Part model, mm, in its own coordinate system. A direction names the side the tool comes from. Give positions to 0.01 mm unless a question says otherwise; leave off trailing zeros. Order: outer loops, then holes, each group sorted by start corner. A loop starts at its lowest first (then second) coordinate and runs counter-clockwise, first axis right, second up. Notation, with made-up numbers: (-4, -10) - (28, -10) arc R19 cw to (28, -5) - close; hole circle Ø2 at (4, 43.5). An arc over 180 degrees is marked (long way). Use a Markdown table: item, result. Add a question column.
from build123d import *

# Parameters (mm, degrees)
BOSS_EXTRUDE1_DEPTH = 152.4
CUT_EXTRUDE1_REACH  = 17.875
SKETCH3_R           = 3.2512
CUT_EXTRUDE2_START  = -275.7932
CUT_EXTRUDE2_DEPTH  = 275.7932
CUT_EXTRUDE3_REACH  = 17.875
SKETCH5_R           = 1.5875


with BuildPart() as part:
    # Sketch2 → Boss-Extrude1 (new body, symmetric)
    with BuildSketch(Plane.XY):
        with BuildLine():
            Line((-7.9375, 0), (7.9375, 0))
            Line((7.9375, 0), (7.9375, 15.875))
            Line((7.9375, 15.875), (7.14375, 15.875))
            ThreePointArc((7.14375, 15.875), (6.582483992, 15.642516008), (6.35, 15.08125))
            Line((6.35, 15.08125), (6.35, 2.38125))
            ThreePointArc((6.35, 2.38125), (6.117516008, 1.819983992), (5.55625, 1.5875))
            Line((5.55625, 1.5875), (-7.14375, 1.5875))
            ThreePointArc((-7.14375, 1.5875), (-7.705016008, 1.355016008), (-7.9375, 0.79375))
            Line((-7.9375, 0.79375), (-7.9375, 0))
        make_face()
    extrude(amount=BOSS_EXTRUDE1_DEPTH, both=True)

    # Sketch3 → Cut-Extrude1 (cut, up to next)
    with BuildSketch(Plane(origin=(7.9375, 0, 0), x_dir=(0, 0, -1), z_dir=(1, 0, 0)), mode=Mode.PRIVATE) as cut_extrude1_sk1:
        with Locations((144.907, 10.7061)):
            Circle(SKETCH3_R)
    cut_extrude1_tool1 = extrude(cut_extrude1_sk1.sketch, amount=-CUT_EXTRUDE1_REACH, mode=Mode.PRIVATE) & part.part
    add(cut_extrude1_tool1.solids().sort_by_distance((7.9375, 10.7061, -144.907))[0], mode=Mode.SUBTRACT)
    # Sketch3 → Cut-Extrude1 (cut, up to next)
    with BuildSketch(Plane(origin=(7.9375, 0, 0), x_dir=(0, 0, -1), z_dir=(1, 0, 0)), mode=Mode.PRIVATE) as cut_extrude1_sk2:
        with Locations((130.9116, 10.7061)):
            Circle(SKETCH3_R)
    cut_extrude1_tool2 = extrude(cut_extrude1_sk2.sketch, amount=-CUT_EXTRUDE1_REACH, mode=Mode.PRIVATE) & part.part
    add(cut_extrude1_tool2.solids().sort_by_distance((7.9375, 10.7061, -130.9116))[0], mode=Mode.SUBTRACT)

    # Sketch4 → Cut-Extrude2 (cut)
    with BuildSketch(Plane.XY.offset(152.4).offset(CUT_EXTRUDE2_START)):
        with BuildLine():
            Line((-7.9375, 0.79375), (-7.9375, 0))
            Line((-7.9375, 0), (7.9375, 0))
            Line((7.9375, 0), (7.9375, 15.875))
            Line((7.9375, 15.875), (7.14375, 15.875))
            ThreePointArc((7.14375, 15.875), (6.582483992, 15.642516008), (6.35, 15.08125))
            Line((6.35, 15.08125), (6.35, 2.38125))
            ThreePointArc((6.35, 2.38125), (6.117516008, 1.819983992), (5.55625, 1.5875))
            Line((5.55625, 1.5875), (-7.14375, 1.5875))
            ThreePointArc((-7.14375, 1.5875), (-7.705016008, 1.355016008), (-7.9375, 0.79375))
        make_face()
    extrude(amount=CUT_EXTRUDE2_DEPTH, mode=Mode.SUBTRACT)

    # Sketch5 → Cut-Extrude3 (cut, up to next)
    with BuildSketch(Plane.XZ, mode=Mode.PRIVATE) as cut_extrude3_sk1:
        with Locations((0, -137.8966)):
            Circle(SKETCH5_R)
    cut_extrude3_tool1 = extrude(cut_extrude3_sk1.sketch, amount=-CUT_EXTRUDE3_REACH, mode=Mode.PRIVATE) & part.part
    add(cut_extrude3_tool1.solids().sort_by_distance((0, 0, -137.8966))[0], mode=Mode.SUBTRACT)


solid = part.part
1. Cut at D-D (y = 6.5). Write the cut outline in (x, z).
2. Tool access for faces 4 (the face through (2, 0, -138)), 5 (the face through (-2, 1.588, -138)): list every direction of +Z, -Z, +X, -X, +Y, -Y with a clear straight run to the whole face (end or side of a thin tool).
3. Cut at A-A (x = 0). Write the cut outline in (y, z), plus the area to 3 significant figures.
4. Pin check, flat tips, straight feed: P1, Ø6, axis at x = 2.5, z = -147, coming from the +Y side; P2, Ø8.5, axis at y = 10.71, z = -144.91, coming from the +X side; P3, Ø8, axis at y = 10.5, z = -126.5, coming from the -X side; P4, Ø1.9, axis at x = 0, z = -137.9, coming from the -Y side (3 decimals). Stop position of each tip, or through.
5. Drill centre lines: probe 1 along Z at (x, y) = (6.75, 10.25); probe 2 along X at (y, z) = (13.75, -140); probe 3 along Y at (x, z) = (2.5, -131.5). Where is each one in solid material? Low to high. Write a range as [from, to].
6. Mould opens along X. For faces 1 (the face through (-0.344, 0.783, -139.446)), 2 (the face through (7.155, 13.448, -132.659)), 3 (the face through (6.35, 9, -138)) say: released by +X, released by -X, zero draft, split by the parting line, or undercut.
Responses:
| question | item | result |
|---|---|---|
| 1 | outline | (6.35, -152.4) - (7.94, -152.4) - (7.94, -123.39) - (6.35, -123.39) - close |
| 2 | face 4 | +Z, -Z, +X, -X, -Y |
| 2 | face 5 | +Z, -Z, -X, +Y |
| 3 | outline | (0, -152.4) - (1.59, -152.4) - (1.59, -139.48) - (0, -139.48) - close; (0, -136.31) - (1.59, -136.31) - (1.59, -123.39) - (0, -123.39) - close |
| 3 | area | 41.0 mm² |
| 4 | P1 | stops at y = 1.59 |
| 4 | P2 | stops at x = 7.94 |
| 4 | P3 | stops at x = 6.35 |
| 4 | P4 | passes through |
| 5 | probe 1 | z = [-152.4, -148.13], [-141.69, -134.13], [-127.69, -123.39] |
| 5 | probe 2 | x = [6.35, 7.94] |
| 5 | probe 3 | y = [0, 1.59] |
| 6 | face 1 | undercut |
| 6 | face 2 | zero draft |
| 6 | face 3 | released by -X |
